Study the drawing (mm; zero at the part's minimum x, y, z) and answer. Round coordinates to 2 decimals unless told otherwise and drop trailing zeros. Loops run counter-clockwise (first coordinate to the right, second up) from the corner with the lowest first, then second, coordinate; pieces in that order, holes last. Notation, with made-up numbers: (15, -19.5) -> (59, -19.5) arc R11 cw to (59, -6.5) -> close; hole circle Ø2 at (-37.5, 35.25). An arc over 180 degrees is marked (long way). Write each question's results on one line, items separated by ' | '. Start each with the question number.
(1) Straight lines are drawn through the part: probe 1 along Y at (x, z) = (5.08, 1.1); probe 2 along X at (y, z) = (6.25, 0.3); probe 3 along Y at (x, z) = (3.5, 1.45). For each, find the intervals that lie inside material, in ascending order.
(2) The part is cut by section A-A (z = 1.2). Determine the outline of the cut face in (x, y), plus the area to 3 significant figures.
(3) Determine the mould class of the marked faces 1, 2, 3 and 4 for opening direction X: released by +X, released by -X, zero draft, split by the parting line, or undercut.
(4) The part is cut by section B-B (y = 7.5). Determine the outline of the cut face in (x, z) (3 decimals).
(5) Flat-ended cylindrical pins translate along their axes: pin 1 (4 mm diameter, centred on x = 22, y = 11, fed in from -Z); pin 2 (3 mm diameter, centred on x = 49.92, y = 7.5, fed in from -Z). Find the tip coordinate at first contact, or state that the pin passes through.
(6) The part is cut by section C-C (x = 49.92). Determine the outline of the cut face in (y, z) (3 decimals), plus the area to 3 significant figures.
(7) The part is cut by section D-D (x = 5). Determine the outline of the cut face in (y, z) (3 decimals).
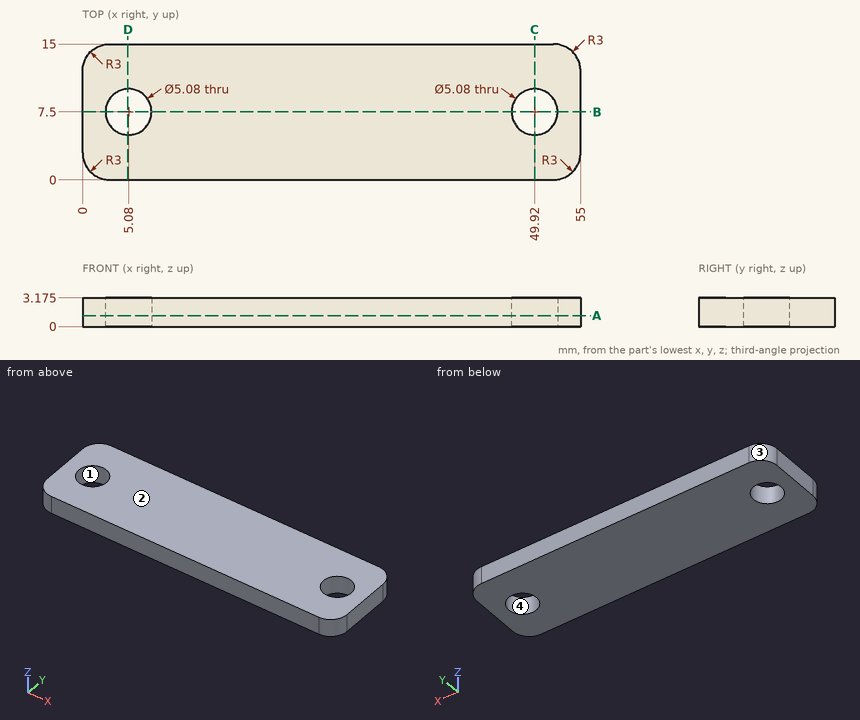
Checked values:
1) probe 1: y = 0 to 4.96, 10.04 to 15 | probe 2: x = 0 to 2.87, 7.29 to 47.71, 52.13 to 55 | probe 3: y = 0 to 5.51, 9.49 to 15
2) outline: (0, 3) arc R3 ccw to (3, 0) -> (52, 0) arc R3 ccw to (55, 3) -> (55, 12) arc R3 ccw to (52, 15) -> (3, 15) arc R3 ccw to (0, 12) -> close; hole circle Ø5.08 at (5.08, 7.5); hole circle Ø5.08 at (49.92, 7.5) | area: 777 mm2
3) face 1: undercut | face 2: zero draft | face 3: released by -X | face 4: undercut
4) outline: (0, 0) -> (2.54, 0) -> (2.54, 3.175) -> (0, 3.175) -> close; (7.62, 0) -> (47.38, 0) -> (47.38, 3.175) -> (7.62, 3.175) -> close; (52.46, 0) -> (55, 0) -> (55, 3.175) -> (52.46, 3.175) -> close
5) pin 1: stops at z = 0 | pin 2: passes through
6) outline: (0, 0) -> (4.96, 0) -> (4.96, 3.175) -> (0, 3.175) -> close; (10.04, 0) -> (15, 0) -> (15, 3.175) -> (10.04, 3.175) -> close | area: 31.5 mm2
7) outline: (0, 0) -> (4.961, 0) -> (4.961, 3.175) -> (0, 3.175) -> close; (10.039, 0) -> (15, 0) -> (15, 3.175) -> (10.039, 3.175) -> close
